```python
from build123d import *

# Parameters (mm, degrees)
SKETCH1_R           = 2.75
SKETCH1_R_2         = 1.5
BOSS_EXTRUDE1_DEPTH = 5
SKETCH2_R           = 4.75
SKETCH2_R_2         = 2.75
BOSS_EXTRUDE2_DEPTH = 35


with BuildPart() as part:
    # Sketch1 → Boss-Extrude1 (new body)
    with BuildSketch(Plane(origin=(0, 0, 0), x_dir=(1, 0, 0), z_dir=(0, 1, 0))):
        with BuildLine():
            Line((-115, 25), (115, 25))
            ThreePointArc((115, 25), (122.071067812, 22.071067812), (125, 15))
            Line((125, 15), (125, -15))
            ThreePointArc((125, -15), (122.071067812, -22.071067812), (115, -25))
            Line((115, -25), (-115, -25))
            ThreePointArc((-115, -25), (-122.071067812, -22.071067812), (-125, -15))
            Line((-125, -15), (-125, 15))
            ThreePointArc((-125, 15), (-122.071067812, 22.071067812), (-115, 25))
        make_face()
        with Locations((90, 0)):
            Circle(SKETCH1_R, mode=Mode.SUBTRACT)
        with Locations((-90, 15)):
            Circle(SKETCH1_R, mode=Mode.SUBTRACT)
        with Locations((-50, 0)):
            Circle(SKETCH1_R, mode=Mode.SUBTRACT)
        with Locations((50, 0)):
            Circle(SKETCH1_R, mode=Mode.SUBTRACT)
        with Locations((-90, -15)):
            Circle(SKETCH1_R, mode=Mode.SUBTRACT)
        with Locations((-100, -20)):
            Circle(SKETCH1_R_2, mode=Mode.SUBTRACT)
        with Locations((100, -20)):
            Circle(SKETCH1_R_2, mode=Mode.SUBTRACT)
    extrude(amount=BOSS_EXTRUDE1_DEPTH)

    # Sketch2 → Boss-Extrude2 (add)
    with BuildSketch(Plane(origin=(0, 0, 0), x_dir=(-1, 0, 0), z_dir=(0, -1, 0))):
        with Locations((90, -15)):
            Circle(SKETCH2_R)
        with Locations((90, -15)):
            Circle(SKETCH2_R_2, mode=Mode.SUBTRACT)
        with Locations((90, 15)):
            Circle(SKETCH2_R)
        with Locations((90, 15)):
            Circle(SKETCH2_R_2, mode=Mode.SUBTRACT)
        with Locations((-90, 0)):
            Circle(SKETCH2_R)
        with Locations((-90, 0)):
            Circle(SKETCH2_R_2, mode=Mode.SUBTRACT)
    extrude(amount=BOSS_EXTRUDE2_DEPTH)


solid = part.part
```
The listing builds one solid part. Answer for the finished solid, in the listing's coordinates (mm). A direction names the side the tool comes from. Coordinates: 2 decimals unless noted, no trailing zeros. Order: outer loops, then holes, each group sorted by start corner. A loop starts at its lowest first (then second) coordinate and runs counter-clockwise, first axis right, second up. Notation, with made-up numbers: M 72,-3.75 L 101,-3.75 A7 ccw 101,9.25 Z; hole C 68,68.5 d5. An arc over 180 degrees is marked long. Answer as a JSON object with one key per item and string values. Group by question number.
1. Section C-C on x = 50 is taken. Write down the section's boundary in (y, z), then the cut area to 4 significant figures.
2. Section B-B on x = -90 is taken. Write down the section's boundary in (y, z).
3. Flat-ended cylindrical pins translate along their axes: P1, Ø7, axis at x = -50, z = 0, coming from the -Y side; P2, Ø9, axis at x = 90, z = 0, coming from the -Y side. Find the tip coordinate at first contact, or state that the pin passes through.
4. A tool of negligible diameter and unlimited length cuts with its end or side. For faces 4 (the flat face through (-93, -35, 15)), 5 (the cylindrical face through (85.47, -17.26, -1.43)), from which of +Z, -Z, +X, -X, +Y, -Y can it reach the whole face along a straight path? Write none if from no direction.
5. Straight lines are drawn through the part: line 1 (Z direction, x = -90, y = 3.2); line 2 (Z direction, x = -90, y = -16.5); line 3 (X direction, y = 3.7, z = 0). For each, find the intervals that lie inside material, in ascending order.
6. Determine the mould class of faces 1 (the cylindrical face through (-121.99, 2.46, 22.15)), 2 (the flat face through (-125, 2, 0)), 3 (the cylindrical face through (-52.747, 2.465, -0.121)) for opening direction Z: released by +Z, released by -Z, zero draft, split by the parting line, or undercut.
7. Section A-A on y = -8 is taken. Write down the section's boundary in (x, z), then the cut area to 3 significant figures.
Values follow:
{
 "1": {"outline": "M 0,-25 L 5,-25 L 5,-2.75 L 0,-2.75 Z; M 0,2.75 L 5,2.75 L 5,25 L 0,25 Z", "area": "222.5 mm2"},
 "2": {"outline": "M -35,-19.75 L 0,-19.75 L 0,-25 L 5,-25 L 5,-17.75 L -35,-17.75 Z; M -35,-12.25 L 5,-12.25 L 5,12.25 L -35,12.25 L -35,10.25 L 0,10.25 L 0,-10.25 L -35,-10.25 Z; M -35,17.75 L 5,17.75 L 5,25 L 0,25 L 0,19.75 L -35,19.75 Z"},
 "3": {"P1": "y = 0", "P2": "y = -35"},
 "4": {"face 4": "+Z, -Z, +X, -X, -Y", "face 5": "-Y"},
 "5": {"line 1": "-25 to -17.75, -12.25 to 12.25, 17.75 to 25", "line 2": "-19.75 to -17.75, -12.25 to -10.25, 10.25 to 12.25, 17.75 to 19.75", "line 3": "-125 to -52.75, -47.25 to 47.25, 52.75 to 87.25, 92.75 to 125"},
 "6": {"face 1": "released by +Z", "face 2": "zero draft", "face 3": "undercut"},
 "7": {"outline": "C -90,-15 d9.5; C -90,15 d9.5; C 90,0 d9.5; hole C -90,-15 d5.5; hole C -90,15 d5.5; hole C 90,0 d5.5", "area": "141 mm2"}
}
